Could you check a few things on this drawing? It's one solid part, dimensions in mm from its lowest x, y, z. Round coordinates to 2 decimals unless told otherwise and drop trailing zeros. Write each loop counter-clockwise with the first axis right and the second up, starting at its lowest first coordinate (ties: lowest second). Pieces come first, ordered by that corner, then holes. Notation, with made-up numbers: M 27.5,-14 L 46.5,-14 A26 ccw 46.5,0 Z; hole C 48,18 d2. An arc over 180 degrees is marked long. One line per item, written item: value. Start each with the question number.
(1) If I drill on L1, parallel to Y at x = 7.5, z = 2.75 (1 decimal); L2, parallel to X at y = 12.5, z = 3.5 (1 decimal); L3, parallel to Y at x = 8, z = 1.5 (1 decimal), over which ranges is the centre line in solid material (lowest first)?
(2) I want a section at A-A on x = 7.5. Please give me the cut outline in (y, z) (1 decimal).
(3) I want a section at B-B on y = 14. Please give me the cut outline in (x, z) (1 decimal).
(4) Thinking about a two-plate mould opening in X: for the marked faces 1, 2, 3 and 4, which applies, released by +X, released by -X, zero draft, split by the parting line, or undercut?
(5) I want a section at D-D on y = 5.5. Please give me the cut outline in (x, z) (1 decimal).
(6) I'm going to push flat-ended pins straight in: pin 1 Ø3 at (y, z) = (3.5, 6) entering from -X; pin 2 Ø2 at (x, y) = (3.5, 15) entering from -Z; pin 3 Ø2 at (y, z) = (13, 5.5) entering from -X. Where does each tip first touch, or does it pass through?
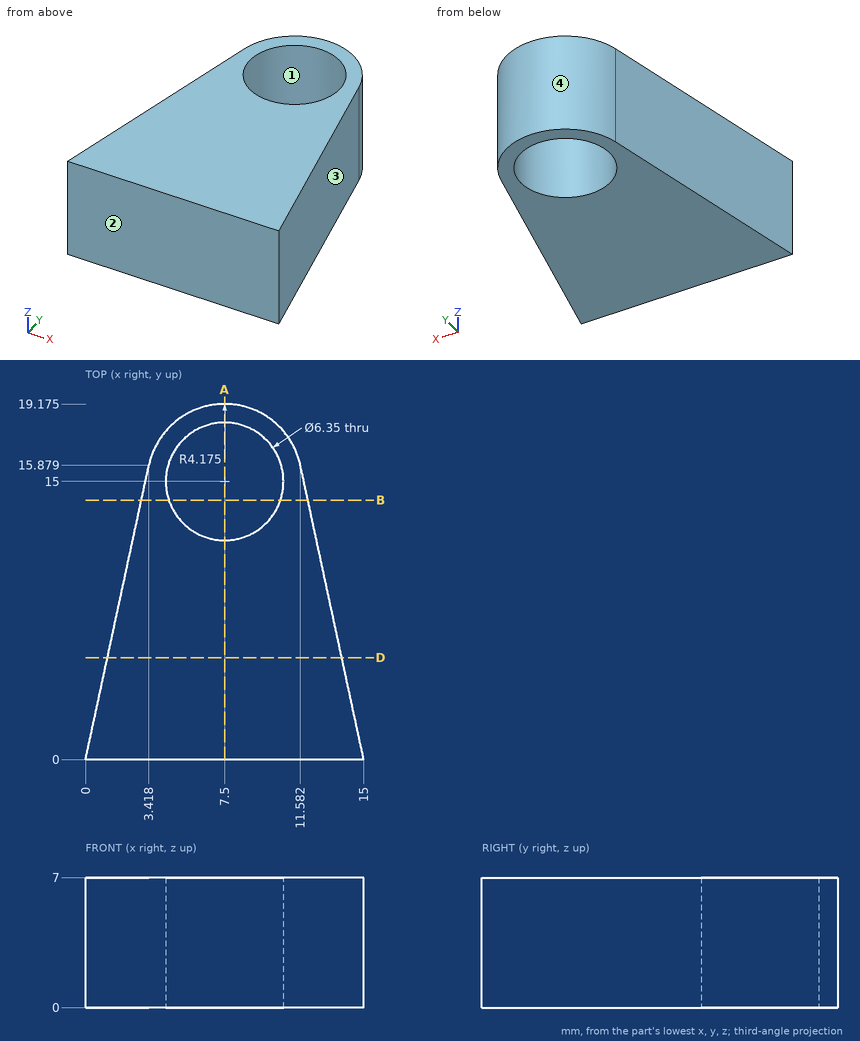
Found:
1. L1: y = 0 to 11.8, 18.2 to 19.2
1. L2: x = 2.7 to 5.5, 9.5 to 12.3
1. L3: y = 0 to 11.9, 18.1 to 19.1
2. outline: M 0,0 L 11.8,0 L 11.8,7 L 0,7 Z; M 18.2,0 L 19.2,0 L 19.2,7 L 18.2,7 Z
3. outline: M 3,0 L 4.5,0 L 4.5,7 L 3,7 Z; M 10.5,0 L 12,0 L 12,7 L 10.5,7 Z
4. face 1: undercut
4. face 2: zero draft
4. face 3: released by +X
4. face 4: split by the parting line
5. outline: M 1.2,0 L 13.8,0 L 13.8,7 L 1.2,7 Z
6. pin 1: stops at x = 0.43
6. pin 2: stops at z = 0
6. pin 3: stops at x = 2.58
